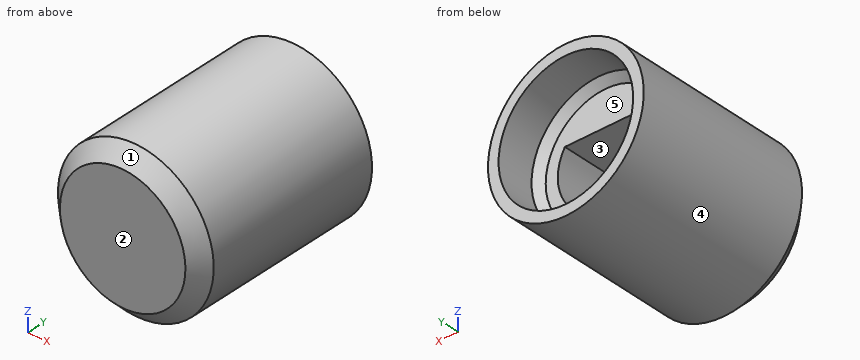
from build123d import *

# Parameters (mm, degrees)
SKETCH1_R           = 5.15
BOSS_EXTRUDE1_DEPTH = 10
SKETCH2_R           = 5.15
BOSS_EXTRUDE2_DEPTH = 2
SKETCH4_R           = 5.15
SKETCH4_R_2         = 4.45
BOSS_EXTRUDE3_DEPTH = 3
CHAMFER1_SIZE       = 1
CHAMFER2_SIZE       = 0.5


with BuildPart() as part:
    # Sketch1 → Boss-Extrude1 (new body)
    with BuildSketch(Plane(origin=(0, 0, 0), x_dir=(1, 0, 0), z_dir=(0, 1, 0))):
        with Locations(Location((0, 0, 0), (0, 0, 270))):
            Circle(SKETCH1_R)
        with BuildLine():
            Line((2.683281573, -1.65), (-2.683281573, -1.65))
            ThreePointArc((-2.683281573, -1.65), (0, 3.15), (2.683281573, -1.65))
        make_face(mode=Mode.SUBTRACT)
    extrude(amount=BOSS_EXTRUDE1_DEPTH)

    # Sketch2 → Boss-Extrude2 (add)
    with BuildSketch(Plane.XZ):
        with Locations(Location((0, 0, 0), (0, 0, 90))):
            Circle(SKETCH2_R)
    extrude(amount=-BOSS_EXTRUDE2_DEPTH)

    # Sketch4 → Boss-Extrude3 (add)
    with BuildSketch(Plane(origin=(0, 10, 0), x_dir=(1, 0, 0), z_dir=(0, 1, 0))):
        with Locations(Location((0, 0, 0), (0, 0, 270))):
            Circle(SKETCH4_R)
        with Locations(Location((0, 0, 0), (0, 0, 270))):
            Circle(SKETCH4_R_2, mode=Mode.SUBTRACT)
    extrude(amount=BOSS_EXTRUDE3_DEPTH)

    # Chamfer1
    chamfer1_edges = [part.edges().sort_by_distance(p)[0] for p in [
        (0, 0, -5.15),
    ]]
    chamfer(chamfer1_edges, length=CHAMFER1_SIZE)

    # Chamfer2
    chamfer2_edges = [part.edges().sort_by_distance(p)[0] for p in [
        (0, 10, -4.45),
    ]]
    chamfer(chamfer2_edges, length=CHAMFER2_SIZE)


solid = part.part
Read the model definition and answer for the solid it produces. Units are mm, in the model's axes. Face numbers are marked on the shaded views. A direction names the side the tool comes from. Round coordinates to 2 decimals unless told otherwise and drop trailing zeros. Loops run counter-clockwise (first coordinate to the right, second up) from the corner with the lowest first, then second, coordinate; pieces in that order, holes last. Notation, with made-up numbers: (-27, -10) - (24, -10) arc R16 ccw to (24, 11) - close; hole circle Ø5 at (-11.75, 44). An arc over 180 degrees is marked (long way). One line per question, with ' | ' between items. Start each with the question number.
Q1. For the marked faces 4 and 5, determine the directions among +Z, -Z, +X, -X, +Y, -Y from which every point of the face is accessible in a straight line to the end or side of a thin tool.
Q2. For a pull along Z with two mould halves and no side action, classify the marked faces 1, 2 and 3 as +Z half, -Z half, draft (parallel to the pull), parting line (faces both ways), or undercut.
Q3. Section D-D on y = 3.5 is taken. Give the vertices of the cut face in (x, z).
Q4. Find the intervals of material crossed by L1, parallel to X at y = 12.2, z = 0; L2, parallel to X at y = 7, z = 0; L3, parallel to Y at x = -2.5, z = -0.5, in increasing order.
Q5. Section A-A on z = 0 is taken. Give the vertices of the cut face in (x, y), plus the area to 4 significant figures.
Q6. Section C-C on y = 1.75 is taken. Give the vertices of the cut face in (x, z), plus the area to 3 significant figures.
Q7. Section B-B on x = 0 is taken. Give the vertices of the cut face in (y, z).
Q8. Flat-ended cylindrical pins translate along their axes: pin 1 (3 mm diameter, centred on y = 4.5, z = -3, fed in from -X); pin 2 (4 mm diameter, centred on x = -1, z = -0.5, fed in from +Y); pin 3 (1.5 mm diameter, centred on y = 5.5, z = -2.5, fed in from -X). Find the tip coordinate at first contact, or state that the pin passes through.
Established:
1) face 4: +Y, -Y | face 5: +Y
2) face 1: parting line | face 2: draft | face 3: undercut
3) outline: circle Ø10.3 at (0, 0); hole (-2.68, 1.65) arc R3.15 ccw (long way) to (2.68, 1.65) - close
4) L1: -5.15 to -4.45, 4.45 to 5.15 | L2: -5.15 to -3.15, 3.15 to 5.15 | L3: 0 to 2
5) outline: (-5.15, 1) - (-4.15, 0) - (4.15, 0) - (5.15, 1) - (5.15, 13) - (4.45, 13) - (4.45, 10.5) - (3.95, 10) - (3.15, 10) - (3.15, 2) - (-3.15, 2) - (-3.15, 10) - (-3.95, 10) - (-4.45, 10.5) - (-4.45, 13) - (-5.15, 13) - close | area: 56.05 mm²
6) outline: circle Ø10.3 at (0, 0) | area: 83.3 mm²
7) outline: (0, -4.15) - (1, -5.15) - (13, -5.15) - (13, -4.45) - (10.5, -4.45) - (10, -3.95) - (10, -3.15) - (2, -3.15) - (2, 1.65) - (10, 1.65) - (10, 3.95) - (10.5, 4.45) - (13, 4.45) - (13, 5.15) - (1, 5.15) - (0, 4.15) - close
8) pin 1: x = -4.93 | pin 2: y = 2 | pin 3: x = -4.84
